```python
from build123d import *

# Parameters (mm, degrees)
SKETCH1_W          = 396.875
SKETCH1_H          = 485.775
EXTRUDE1_DEPTH     = 165.1
FILLET1_R          = 12.7
FILLET2_R          = 12.7
SHELL1_T           = -1.6002
SKETCH2_R          = 28.575
SKETCH2_R_2        = 2.5527
CUT_EXTRUDE1_DEPTH = 25.4
SKETCH6_R          = 3.4544
CUT_EXTRUDE5_DEPTH = 551.102537743
SKETCH7_R          = 1.9812
CUT_EXTRUDE6_DEPTH = 551.102537743
CUT_EXTRUDE7_REACH = 650.649
SKETCH8_R          = 2.0447


with BuildPart() as part:
    # Sketch1 → Extrude1 (new body)
    with BuildSketch(Plane(origin=(0, 0, 0), x_dir=(1, 0, 0), z_dir=(0, 1, 0))):
        with Locations((0, 242.8875)):
            Rectangle(SKETCH1_W, SKETCH1_H)
    extrude(amount=EXTRUDE1_DEPTH)

    # Fillet1
    fillet1_edges = [part.edges().sort_by_distance(p)[0] for p in [
        (-198.4375, 82.55, -485.775),
        (198.4375, 82.55, -485.775),
        (198.4375, 82.55, 0),
        (-198.4375, 82.55, 0),
    ]]
    fillet(fillet1_edges, radius=FILLET1_R)

    # Fillet2
    fillet2_edges = [part.edges().sort_by_distance(p)[0] for p in [
        (0, 0, 0),
        (-198.4375, 0, -242.8875),
        (0, 0, -485.775),
        (198.4375, 0, -242.8875),
        (194.717756121, 0, -3.719743879),
        (194.717756121, 0, -482.055256121),
        (-194.717756121, 0, -482.055256121),
        (-194.717756121, 0, -3.719743879),
    ]]
    fillet(fillet2_edges, radius=FILLET2_R)

    # Shell1
    shell1_openings = [part.faces().sort_by_distance(p)[0] for p in [
        (0, 165.1, -242.8875),
    ]]
    offset(amount=SHELL1_T, openings=shell1_openings, kind=Kind.INTERSECTION)

    # Sketch2 → Cut-Extrude1 (cut)
    with BuildSketch(Plane.XY):
        with Locations((-44.45, 47.625)):
            Circle(SKETCH2_R)
        with Locations(Location((44.45, 47.625, 0), (0, 0, 180))):
            Circle(SKETCH2_R)
        with Locations((-92.075, 84.1502)):
            Circle(SKETCH2_R_2)
        with Locations((-92.075, 19.05)):
            Circle(SKETCH2_R_2)
        with Locations(Location((92.075, 19.05, 0), (0, 0, 180))):
            Circle(SKETCH2_R_2)
        with Locations(Location((92.075, 84.1502, 0), (0, 0, 180))):
            Circle(SKETCH2_R_2)
        with Locations((0, 84.1502)):
            Circle(SKETCH2_R_2)
        with Locations((0, 19.05)):
            Circle(SKETCH2_R_2)
        with Locations((-177.8, 84.1502)):
            Circle(SKETCH2_R_2)
        with Locations(Location((177.8, 84.1502, 0), (0, 0, 180))):
            Circle(SKETCH2_R_2)
    extrude(amount=-CUT_EXTRUDE1_DEPTH, mode=Mode.SUBTRACT)

    # Sketch6 → Cut-Extrude5 (cut, through all)
    with BuildSketch(Plane(origin=(0, 0, 0), x_dir=(1, 0, 0), z_dir=(0, 1, 0))):
        with Locations(Location((0, 457.2, 0), (0, 0, 270))):
            Circle(SKETCH6_R)
    extrude(amount=CUT_EXTRUDE5_DEPTH, mode=Mode.SUBTRACT)

    # Sketch7 → Cut-Extrude6 (cut, through all)
    with BuildSketch(Plane(origin=(0, 0, 0), x_dir=(1, 0, 0), z_dir=(0, 1, 0))):
        with Locations(Location((-60.325, 103.2002, 0), (0, 0, 270))):
            Circle(SKETCH7_R)
        with Locations(Location((-60.325, 369.8748, 0), (0, 0, 270))):
            Circle(SKETCH7_R)
        with Locations(Location((60.325, 369.8748, 0), (0, 0, 90))):
            Circle(SKETCH7_R)
        with Locations(Location((60.325, 103.2002, 0), (0, 0, 90))):
            Circle(SKETCH7_R)
    extrude(amount=CUT_EXTRUDE6_DEPTH, mode=Mode.SUBTRACT)

    # Sketch8 → Cut-Extrude7 (cut, up to next)
    with BuildSketch(Plane(origin=(198.4375, 0, 0), x_dir=(0, 0, -1), z_dir=(1, 0, 0)), mode=Mode.PRIVATE) as cut_extrude7_sk1:
        with Locations((242.8875, 127.762)):
            Circle(SKETCH8_R)
    cut_extrude7_tool1 = extrude(cut_extrude7_sk1.sketch, amount=-CUT_EXTRUDE7_REACH, mode=Mode.PRIVATE) & part.part
    # Sketch8 → Cut-Extrude7 (cut, up to next)
    with BuildSketch(Plane(origin=(198.4375, 0, 0), x_dir=(0, 0, -1), z_dir=(1, 0, 0)), mode=Mode.PRIVATE) as cut_extrude7_sk2:
        with Locations((242.8875, 107.8484)):
            Circle(SKETCH8_R)
    cut_extrude7_tool2 = extrude(cut_extrude7_sk2.sketch, amount=-CUT_EXTRUDE7_REACH, mode=Mode.PRIVATE) & part.part
    cut_extrude7_1 = cut_extrude7_tool1.solids().sort_by_distance((198.4375, 127.762, -242.8875))[0]
    add(cut_extrude7_1, mode=Mode.SUBTRACT)
    cut_extrude7_2 = cut_extrude7_tool2.solids().sort_by_distance((198.4375, 107.8484, -242.8875))[0]
    add(cut_extrude7_2, mode=Mode.SUBTRACT)
    cut_extrude7 = cut_extrude7_1 + cut_extrude7_2  # Cut-Extrude7 as one shape, for the pattern or mirror that repeats it

    # Mirror1: Cut-Extrude7 across plane
    add(cut_extrude7.mirror(Plane(origin=(0, 0, 0), x_dir=(0, 0, 1), z_dir=(1, 0, 0))), mode=Mode.SUBTRACT)


solid = part.part
```
Work out the finished part from the listing and answer in its coordinate system (mm). A direction names the side the tool comes from. Coordinates: 2 decimals unless noted, no trailing zeros. Write each loop counter-clockwise with the first axis right and the second up, starting at its lowest first coordinate (ties: lowest second). Pieces come first, ordered by that corner, then holes.
Q1. Determine the mould class of faces 1 (the face through (-198.438, 88, -240)), 2 (the face through (-3, 88, 0)), 3 (the face through (-193.499, 4.765, -239.665)) for opening direction X: released by +X, released by -X, zero draft, split by the parting line, or undercut.
Q2. Find the intervals of material crossed by line 1 (X direction, y = 104, z = -220); line 2 (Z direction, x = -24, y = 24) (3 decimals); line 3 (Z direction, x = -22, y = 52) (3 decimals), in increasing order.
Q3. Which of the six approach directions +Z, -Z, +X, -X, +Y, -Y give full straight-line access (tool end or side, diameter ignored) to faces 4 (the face through (-2.6, 4.77, -480.84)), 5 (the face through (194.618, 3.622, -246.11))?
Q4. A cutting plane is placed at C-C, the plane y = 53. Give the vertices of the cut face in (x, z) (1 decimal).
Q5. A cutting plane is placed at A-A, the plane x = -44.45. Give the vertices of the cut face in (y, z) (3 decimals), then the cut area to 3 significant figures.
Q6. A cutting plane is placed at B-B, the plane z = -441.5. Give the vertices of the cut face in (x, y), then the cut area to 3 significant figures.
Q7. A cutting plane is placed at D-D, the plane x = -169.5. Give the vertices of the cut face in (y, z) (3 decimals), then the cut area to 3 significant figures.
Q8. Each of these flat-tipped pins is pushed along its axis until it touches: pin 1 Ø2.5 at (y, z) = (127.76, -242.89) entering from -X; pin 2 Ø1 at (x, y) = (50.5, 57) entering from +Z; pin 3 Ø6.5 at (x, z) = (60.32, -369.87) entering from +Y. Where does it stop, or does it pass through?
Findings below:
1. face 1: released by -X
1. face 2: zero draft
1. face 3: undercut
2. line 1: x = -198.44 to -196.84, 196.84 to 198.44
2. line 2: z = -485.775 to -484.175, -1.6 to 0
2. line 3: z = -485.775 to -484.175
3. face 4: +Y
3. face 5: +Z, -Z, +X, -Y
4. outline: (-198.4, -473.1) arc R12.7 ccw to (-185.7, -485.8) - (185.7, -485.8) arc R12.7 ccw to (198.4, -473.1) - (198.4, -12.7) arc R12.7 ccw to (185.7, 0) - (72.5, 0) - (72.5, -1.6) - (185.7, -1.6) arc R11.1 cw to (196.8, -12.7) - (196.8, -473.1) arc R11.1 cw to (185.7, -484.2) - (-185.7, -484.2) arc R11.1 cw to (-196.8, -473.1) - (-196.8, -12.7) arc R11.1 cw to (-185.7, -1.6) - (-72.5, -1.6) - (-72.5, 0) - (-185.7, 0) arc R12.7 ccw to (-198.4, -12.7) - close; (-16.4, -1.6) - (16.4, -1.6) - (16.4, 0) - (-16.4, 0) - close
5. outline: (0, -473.075) arc R12.7 ccw to (12.7, -485.775) - (165.1, -485.775) - (165.1, -484.175) - (12.7, -484.175) arc R11.1 cw to (1.6, -473.075) - (1.6, -12.7) arc R11.1 cw to (12.7, -1.6) - (19.05, -1.6) - (19.05, 0) - (12.7, 0) arc R12.7 ccw to (0, -12.7) - close; (76.2, -1.6) - (165.1, -1.6) - (165.1, 0) - (76.2, 0) - close
5. area: 1,190 mm2
6. outline: (-198.44, 12.7) arc R12.7 ccw to (-185.74, 0) - (185.74, 0) arc R12.7 ccw to (198.44, 12.7) - (198.44, 165.1) - (196.84, 165.1) - (196.84, 12.7) arc R11.1 cw to (185.74, 1.6) - (-185.74, 1.6) arc R11.1 cw to (-196.84, 12.7) - (-196.84, 165.1) - (-198.44, 165.1) - close
6. area: 1,140 mm2
7. outline: (0, -473.075) arc R12.7 ccw to (12.7, -485.775) - (165.1, -485.775) - (165.1, -484.175) - (12.7, -484.175) arc R11.1 cw to (1.6, -473.075) - (1.6, -12.7) arc R11.1 cw to (12.7, -1.6) - (165.1, -1.6) - (165.1, 0) - (12.7, 0) arc R12.7 ccw to (0, -12.7) - close
7. area: 1,280 mm2
8. pin 1: passes through
8. pin 2: stops at z = -484.17
8. pin 3: stops at y = 1.6
